from build123d import *

# Parameters (mm, degrees)
F0_W        = 60.96
F0_H        = 104.14
F1_DEPTH    = 7.62
F2_W        = 45.9153815961
F2_H        = 38.1
F2_R        = 17.78
F2_R_2      = 7.62
F3_DEPTH    = 0.254
F4_W        = 13.0856782198
F4_H        = 1.975195948
F5_DEPTH    = 2.54
F6_R        = 2.2527466913
F7_DEPTH    = 2.54
F8_T1_DEPTH = 33.02
F9_W        = 32.8376358375
F9_H        = 1.8517468125
F10_DEPTH   = 2.54


# Not quite as in the source:
# - a fillet or chamfer that OpenCascade refuses, or shapes differently, is made with other operations: its cross-section is extruded or revolved along the edge and cut away or added


with BuildPart() as f1:
    # F0 (on Front) → F1 (new body)
    with BuildSketch(Plane.XZ):
        with Locations((-22.7986111199, 3.2297596335)):
            Rectangle(F0_W, F0_H)
    extrude(amount=F1_DEPTH)

    # F2 (on face) → F3 (join)
    with BuildSketch(Plane.XZ.offset(7.62)):
        with Locations((-23.1955593918, 27.3597596335)):
            Rectangle(F2_W, F2_H)
        with Locations((-22.7986111199, -25.5444776267)):
            Circle(F2_R)
        with Locations((-22.7986111199, -25.5444776267)):
            Circle(F2_R_2, mode=Mode.SUBTRACT)
    extrude(amount=F3_DEPTH)

    # F4 (on face) → F5 (cut)
    with BuildSketch(Plane(origin=(0, 0, -48.8402403665), x_dir=(1, 0, 0), z_dir=(0, 0, -1))):
        with Locations((-44.3373024464, 3.3156641293)):
            Rectangle(F4_W, F4_H)
    extrude(amount=-F5_DEPTH, mode=Mode.SUBTRACT)

    # F6 (on face) → F7 (cut)
    with BuildSketch(Plane(origin=(0, 0, -48.8402403665), x_dir=(1, 0, 0), z_dir=(0, 0, -1))):
        with Locations((-1.6869211104, 4.2321491055)):
            Circle(F6_R)
    extrude(amount=-F7_DEPTH, mode=Mode.SUBTRACT)

    # F8: fillet of radius 5.08 on 4 edges, made by hand

    # F8_s2 → F8_t1 (cut)
    with BuildSketch(Plane.XZ.offset(-12.7)):
        with BuildLine():
            ThreePointArc((2.6013888801, 55.2997596335), (6.1934913285, 53.811862082), (7.6813888801, 50.2197596335))
            Line((7.6813888801, 50.2197596335), (7.6813888801, 55.2997596335))
            Line((7.6813888801, 55.2997596335), (2.6013888801, 55.2997596335))
        make_face()
        with BuildLine():
            ThreePointArc((-48.1986111199, 55.2997596335), (-51.7907135683, 53.811862082), (-53.2786111199, 50.2197596335))
            Line((-53.2786111199, 50.2197596335), (-53.2786111199, 55.2997596335))
            Line((-53.2786111199, 55.2997596335), (-48.1986111199, 55.2997596335))
        make_face()
        with BuildLine():
            ThreePointArc((7.6813888801, -43.7602403665), (6.1934913285, -47.3523428149), (2.6013888801, -48.8402403665))
            Line((2.6013888801, -48.8402403665), (7.6813888801, -48.8402403665))
            Line((7.6813888801, -48.8402403665), (7.6813888801, -43.7602403665))
        make_face()
        with BuildLine():
            ThreePointArc((-53.2786111199, -43.7602403665), (-51.7907135683, -47.3523428149), (-48.1986111199, -48.8402403665))
            Line((-48.1986111199, -48.8402403665), (-53.2786111199, -48.8402403665))
            Line((-53.2786111199, -48.8402403665), (-53.2786111199, -43.7602403665))
        make_face()
    extrude(amount=F8_T1_DEPTH, mode=Mode.SUBTRACT)

    # F9 (on face) → F10 (cut)
    with BuildSketch(Plane.XY.offset(55.2997596335)):
        with Locations((-22.7386062033, -4.1089197621)):
            Rectangle(F9_W, F9_H)
    extrude(amount=-F10_DEPTH, mode=Mode.SUBTRACT)


solid = f1.part
CAD build for the part. Positions are in the model's coordinates, mm. A direction names the side the tool comes from. Round coordinates to 2 decimals unless told otherwise and drop trailing zeros. Loops run counter-clockwise (first coordinate to the right, second up) from the corner with the lowest first, then second, coordinate; pieces in that order, holes last.
(1) Cut at A-A (x = -33). Give the cut face in (y, z).
(2) Cut at B-B (z = -15). Give the cut face in (x, y).
(3) Drop flat-ended pins along their axis: pin 1 (2 mm diameter, centred on x = -44.5, z = -48, fed in from -Y); pin 2 (0.9 mm diameter, centred on x = -16, y = -4.5, fed in from +Z); pin 3 (0.6 mm diameter, centred on y = -3.5, z = -47.5, fed in from -X). Give the stop position or say it passes through.
(4) Two-plate mould, pull along Y, no slides. Class faces 6 (the flat face through (-24, -7.874, 28)), 7 (the cylindrical face through (6.233, -3.757, -47.313)), 8 (the flat face through (-37.794, -3, -48)): +Y half, -Y half, draft (parallel to the pull), parting line (faces both ways), or undercut.
(5) Which spindle directions (+Z, -Z, +X, -X, +Y, -Y) get a long thin tool onto all of the face, cutting with end or side? Do faces 1 (the flat face through (-23, 0, 4)), 2 (the flat face through (-2, -4, -46.3)), 3 (the cylindrical face through (6.154, -3.757, 53.851)), 4 (the flat face through (-6.32, -4, 54)), 5 (the flat face through (-23, -7.62, -25)). Say none if no direction does.
(6) Cut at C-C (x = -25). Give the cut face in (y, z).
(7) Wall check: line 1 along Z through (x, y) = (-42, -4); line 2 along Z through (x, y) = (-18, -3.75); line 3 along Y through (x, z) = (-31.5, 7). Give the ranges that are in metal, low to high.
Findings below:
1. outline: (-7.87, -40.11) - (-7.62, -40.11) - (-7.62, -48.84) - (0, -48.84) - (0, 55.3) - (-3.18, 55.3) - (-3.18, 52.76) - (-5.03, 52.76) - (-5.03, 55.3) - (-7.62, 55.3) - (-7.62, 46.41) - (-7.87, 46.41) - (-7.87, 8.31) - (-7.62, 8.31) - (-7.62, -10.98) - (-7.87, -10.98) - close
2. outline: (-53.28, -7.62) - (-37.11, -7.62) - (-37.11, -7.87) - (-8.48, -7.87) - (-8.48, -7.62) - (7.68, -7.62) - (7.68, 0) - (-53.28, 0) - close
3. pin 1: stops at y = -7.62
3. pin 2: stops at z = 52.76
3. pin 3: stops at x = -51.94
4. face 6: -Y half
4. face 7: draft
4. face 8: undercut
5. face 1: +Z, -Z, +X, -X, +Y
5. face 2: -Z
5. face 3: +Z, +X, +Y, -Y
5. face 4: +Z
5. face 5: -Y
6. outline: (-7.87, -43.19) - (-7.62, -43.19) - (-7.62, -48.84) - (0, -48.84) - (0, 55.3) - (-3.18, 55.3) - (-3.18, 52.76) - (-5.03, 52.76) - (-5.03, 55.3) - (-7.62, 55.3) - (-7.62, 46.41) - (-7.87, 46.41) - (-7.87, 8.31) - (-7.62, 8.31) - (-7.62, -7.9) - (-7.87, -7.9) - (-7.87, -18.25) - (-7.62, -18.25) - (-7.62, -32.84) - (-7.87, -32.84) - close
7. line 1: z = -46.3 to 55.3
7. line 2: z = -48.84 to 52.76
7. line 3: y = -7.62 to 0
